Check sheet for the modelled part. Datum: model origin and axes. Units: mm. Round coordinates to 2 decimals unless told otherwise and drop trailing zeros. Order: outer loops, then holes, each group sorted by start corner. A loop starts at its lowest first (then second) coordinate and runs counter-clockwise, first axis right, second up. Notation, with made-up numbers: (82, -20.5) -> (88, -20.5) arc R31 cw to (88, 10.5) -> close; hole circle Ø8 at (89.5, 47.25). An arc over 180 degrees is marked (long way). Answer in a Markdown table with one row per item. Add a question column.
1. Material ranges on L1, parallel to Y at x = 38, z = 1.9; L2, parallel to X at y = -19.5, z = 2.75; L3, parallel to X at y = 12.5, z = 2.9, recorded low to high. Write a range as from..to.
2. Sectioned sample at D-D, the plane x = 26.5. Record the boundary of the cut face in (y, z) (3 decimals).
3. Sectioned sample at B-B, the plane z = 0.95. Record the boundary of the cut face in (x, y) (3 decimals), then the cut area to 3 significant figures.
4. Depth check by flat-ended pin: P1, Ø5.5, axis at x = 5.08, y = 55.63, coming from the -Z side. Enter the tip coordinate at first touch or a pass-through.
5. Sectioned sample at C-C, the plane y = 37.5. Record the boundary of the cut face in (x, z) (3 decimals).
6. Sectioned sample at A-A, the plane x = 38. Record the boundary of the cut face in (y, z) (3 decimals).
```python
from build123d import *

# Parameters (mm, degrees)
SKETCH1_R           = 1.65
SKETCH1_R_2         = 2
BOSS_EXTRUDE1_DEPTH = 3.175


with BuildPart() as part:
    # Sketch1 → Boss-Extrude1 (new body)
    with BuildSketch(Plane(origin=(0, 0, 0), x_dir=(-1, 0, 0), z_dir=(0, 0, 1))):
        with BuildLine():
            Line((0, -62.136729163), (0, 62.869580678))
            ThreePointArc((0, 62.869580678), (-48.575, 0.366425758), (0, -62.136729163))
        make_face()
        with Locations((-5.075, 56.366425758)):
            Circle(SKETCH1_R, mode=Mode.SUBTRACT)
        with Locations((-21.638471196, 46.366425758)):
            Circle(SKETCH1_R, mode=Mode.SUBTRACT)
        with Locations((-5.075, -55.633574242)):
            Circle(SKETCH1_R, mode=Mode.SUBTRACT)
        with Locations((-21.638471196, -45.633574242)):
            Circle(SKETCH1_R, mode=Mode.SUBTRACT)
        with Locations((-38, 20.287222228)):
            Circle(SKETCH1_R_2, mode=Mode.SUBTRACT)
        with Locations((-38.301731617, -19.711639731)):
            Circle(SKETCH1_R_2, mode=Mode.SUBTRACT)
    extrude(amount=BOSS_EXTRUDE1_DEPTH)


solid = part.part
```
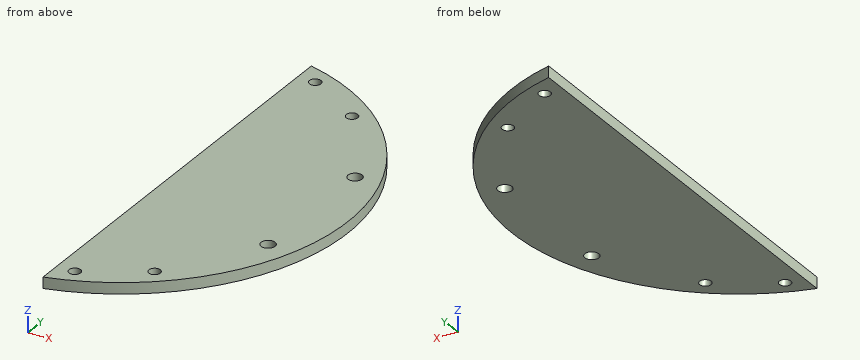
Answer key:
| question | item | result |
|---|---|---|
| 1 | L1 | y = -35.75..-22.29, -18.29..17.73, 21.69..35.02 |
| 1 | L2 | x = 0..36.16, 39.84..45.67 |
| 1 | L3 | x = 0..47.28 |
| 2 | outline | (-48.95, 0) -> (48.217, 0) -> (48.217, 3.175) -> (-48.95, 3.175) -> close |
| 3 | outline | (0, -62.87) arc R64.5 ccw to (0, 62.137) -> close; hole circle Ø3.3 at (5.075, -56.366); hole circle Ø3.3 at (5.075, 55.634); hole circle Ø3.3 at (21.638, -46.366); hole circle Ø3.3 at (21.638, 45.634); hole circle Ø4 at (38, -20.287); hole circle Ø4 at (38.302, 19.712) |
| 3 | area | 4,440 mm² |
| 4 | P1 | stops at z = 0 |
| 5 | outline | (0, 0) -> (36.29, 0) -> (36.29, 3.175) -> (0, 3.175) -> close |
| 6 | outline | (-35.755, 0) -> (-22.287, 0) -> (-22.287, 3.175) -> (-35.755, 3.175) -> close; (-18.287, 0) -> (17.735, 0) -> (17.735, 3.175) -> (-18.287, 3.175) -> close; (21.689, 0) -> (35.022, 0) -> (35.022, 3.175) -> (21.689, 3.175) -> close |
